Could you check a few things on this model? Use its own coordinates, in mm. Face numbers are marked on the shaded views. A direction names the side the tool comes from. Coordinates: 2 decimals unless noted, no trailing zeros. Write each loop counter-clockwise with the first axis right and the second up, starting at its lowest first coordinate (ties: lowest second). Pieces come first, ordered by that corner, then holes.
Item 1: For P1, Ø2, axis at x = -23.5, z = 6.5, coming from the -Y side; P2, Ø6, axis at y = 14.5, z = 11.5, coming from the -X side; P3, Ø8, axis at x = -9.5, z = 7, coming from the -Y side, each with a flat end and sliding along its axis, tell me the tip position at first contact or that it passes through.
Item 2: If I drill on probe 1 along X at (y, z) = (0, 16); probe 2 along Z at (x, y) = (-27.5, 4.5), over which ranges is the centre line in solid material (lowest first)?
Item 3: Which directions (+Z, -Z, +X, -X, +Y, -Y) give clear straight access to the entire face, cutting with the end or side of a thin tool? Please do the marked faces 1 and 2.
Item 4: Thinking about a two-plate mould opening in Y: for the marked faces 3, 4 and 5, which applies, +Y half, -Y half, draft (parallel to the pull), parting line (faces both ways), or undercut?
Item 5: I want a section at C-C on z = 27. Please give me the cut outline in (x, y).
Item 6: I want a section at D-D on y = -18.5. Please give me the cut outline in (x, z).
Item 7: I want a section at B-B on x = 0. Please give me the cut outline in (y, z), then the cut area to 3 significant figures.
Item 8: I want a section at A-A on y = 0. Please give me the cut outline in (x, z), then the cut area to 3 significant figures.
from build123d import *

# Parameters (mm, degrees)
F1_R          = 32.5
F2_DEPTH      = 35
F0_R          = 28.5
F3_DEPTH      = 28
F4_W          = 20
F4_H          = 1
F5_DEPTH      = 40
F5_DEPTH_BACK = 33.5


with BuildPart() as f2:
    # F1 (on Top) → F2 (new body)
    with BuildSketch(Plane.XY):
        Circle(F1_R)
    extrude(amount=F2_DEPTH)

    # F0 (on Top) → F3 (cut)
    with BuildSketch(Plane.XY):
        Circle(F0_R)
    extrude(amount=F3_DEPTH, mode=Mode.SUBTRACT)

    # F4 (on Right) → F5 (cut, two sides)
    with BuildSketch(Plane.YZ) as f5_sk:
        with Locations((-4.7494247556, 14.8)):
            Rectangle(F4_W, F4_H)
    extrude(amount=-F5_DEPTH, mode=Mode.SUBTRACT)
    extrude(f5_sk.sketch, amount=F5_DEPTH_BACK, mode=Mode.SUBTRACT)


solid = f2.part
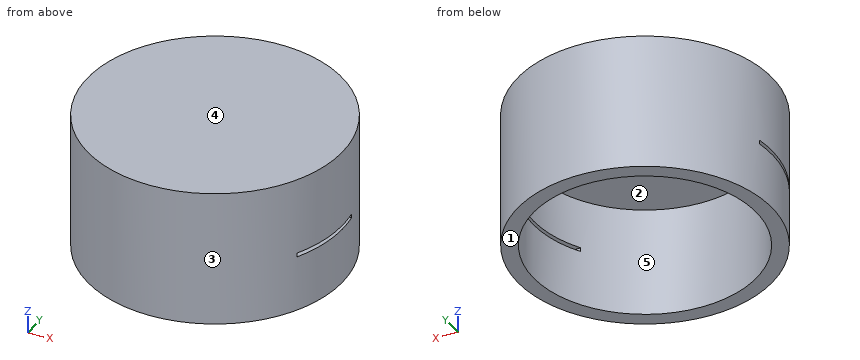
Response values:
1. P1: stops at y = -23.45
1. P2: stops at x = -30.4
1. P3: stops at y = -32.03
2. probe 1: x = -32.5 to -28.5, 28.5 to 32.5
2. probe 2: z = 28 to 35
3. face 1: -Z, +X, -X, +Y, -Y
3. face 2: -Z
4. face 3: parting line
4. face 4: draft
4. face 5: undercut
5. outline: circle Ø65 at (0, 0); hole circle Ø57 at (0, 0)
6. outline: (-26.72, 0) - (-21.68, 0) - (-21.68, 28) - (21.68, 28) - (21.68, 0) - (26.72, 0) - (26.72, 35) - (-26.72, 35) - close
7. outline: (-32.5, 0) - (-28.5, 0) - (-28.5, 28) - (28.5, 28) - (28.5, 0) - (32.5, 0) - (32.5, 35) - (-32.5, 35) - close
7. area: 679 mm2
8. outline: (-32.5, 0) - (-28.5, 0) - (-28.5, 14.3) - (-32.5, 14.3) - close; (-32.5, 15.3) - (-28.5, 15.3) - (-28.5, 28) - (28.5, 28) - (28.5, 15.3) - (32.5, 15.3) - (32.5, 35) - (-32.5, 35) - close; (28.5, 0) - (32.5, 0) - (32.5, 14.3) - (28.5, 14.3) - close
8. area: 671 mm2
